Autodesk Inventor part; units mm, degrees
ref_plane "YZ Plane" through (0, 0, 0) normal (1, 0, 0) x (0, 1, 0)
ref_plane "XZ Plane" through (0, 0, 0) normal (0, 1, 0) x (-1, 0, 0)
ref_plane "XY Plane" through (0, 0, 0) normal (0, 0, 1) x (1, 0, 0)
sketch "Esquisse1" plane through (0, 0, 0) normal (0, 1, 0) x (-1, 0, 0)
  line L0 (-46.5, 50) -> (46.5, 50)
  line L1 (46.5, 50) -> (46.5, -50)
  line L2 (46.5, -50) -> (-46.5, -50)
  line L3 (-46.5, -50) -> (-46.5, 50)
  line L4 (-46.5, 50) -> (46.5, -50) construction
  line L5 (46.5, 50) -> (-46.5, -50) construction
  point P0 (0, 0)
  dimension "d0" = 100
  dimension "d1" = 93
extrude "Extrusion1" add sketch "Esquisse1" along normal blind 88
sketch "Esquisse2" plane through (0, 0, 0) normal (0, -1, 0) x (1, 0, 0)
  line L0 (-43.5, 47) -> (43.5, 47)
  line L1 (43.5, 47) -> (43.5, -47)
  line L2 (43.5, -47) -> (-43.5, -47)
  line L3 (-43.5, -47) -> (-43.5, 47)
  line L4 (-43.5, 47) -> (43.5, -47) construction
  line L5 (43.5, 47) -> (-43.5, -47) construction
  line L6 (46.5, 50) -> (46.5, -50)
  line L7 (-46.5, 50) -> (46.5, 50)
  point P0 (0, 0)
  dimension "d4" = 3
  dimension "d5" = 3
extrude "Extrusion2" cut sketch "Esquisse2" against normal blind 85
sketch "Esquisse3" plane through (-46.5, 0, 50) normal (0, 0, 1) x (1, 0, 0)
  line L0 (0, 88) -> (93, 88)
  line L1 (93, 88) -> (78, 88)
  line L2 (78, 88) -> (78, 73)
  line L3 (78, 73) -> (93, 73)
  line L4 (93, 73) -> (93, 88)
  point P0 (46.5, 0)
  dimension "d8" = 15
  dimension "d9" = 15
extrude "Extrusion3" cut sketch "Esquisse3" against normal up to surface (100 mm away)
sketch "Esquisse4" plane through (-46.5, 0, 50) normal (0, 0, 1) x (1, 0, 0)
  circle A0 centre (73, 68) radius 1.75
  circle A1 centre (33, 68) radius 1.75
  circle A2 centre (73, 30) radius 1.75
  circle A3 centre (33, 30) radius 1.75
  line L0 (93, 0) -> (93, 73)
  line L1 (0, 88) -> (78, 88)
  point P0 (46.5, 0)
  dimension "d12" = 40
  dimension "d13" = 3.5
  dimension "d14" = 3.5
  dimension "d15" = 3.5
  dimension "d16" = 3.5
  dimension "d17" = 40
  dimension "d18" = 0
  dimension "d19" = 0
  dimension "d20" = 38
  dimension "d21" = 20
  dimension "d22" = 20
  dimension "d23" = 0
extrude "Extrusion4" cut sketch "Esquisse4" against normal up to surface (3 mm away)
sketch "Esquisse5" plane through (46.5, 0, -50) normal (0, 0, -1) x (-1, 0, 0)
  circle A0 centre (66.8, 77) radius 2.1
  circle A1 centre (41.4, 77) radius 2.1
  circle A2 centre (11, 44.9) radius 2.1
  circle A3 centre (11, 7.4) radius 2.1
  line L0 (0, 0) -> (0, 73)
  line L1 (15, 88) -> (93, 88)
  line L2 (15, 88) -> (15, 73)
  line L3 (15, 73) -> (0, 73)
  circle A4 centre (83, 7.4) radius 2.1
  line L4 (93, 0) -> (93, 88)
  point P0 (46.5, 0)
  dimension "d26" = 4.2
  dimension "d27" = 4.2
  dimension "d28" = 4.2
  dimension "d29" = 4.2
  dimension "d30" = 11
  dimension "d31" = 0
  dimension "d32" = 11
  dimension "d33" = 0
  dimension "d34" = 37.5
  dimension "d35" = 25.4
  dimension "d36" = 26.4
  dimension "d37" = 28.1
  dimension "d38" = 4.2
  dimension "d39" = 0
  dimension "d40" = 10
extrude "Extrusion5" add sketch "Esquisse5" along normal blind 5.7
sketch "Esquisse6" plane through (-36.5, 7.4, -55.7) normal (0, 0, -1) x (-1, 0, 0)
  point P0 (-36.5, -7.4)
sketch "Esquisse7" plane through (-46.5, 0, 50) normal (0, 0, 1) x (1, 0, 0)
  line L0 (0, 88) -> (78, 88)
  line L1 (65, 88) -> (40, 88)
  line L2 (40, 88) -> (40, 79)
  line L3 (40, 79) -> (65, 79)
  line L4 (65, 79) -> (65, 88)
  line L5 (78, 73) -> (78, 88)
  point P0 (46.5, 0)
  point P1 (78, 80.5)
  point P2 (65, 83.5)
  dimension "d43" = 25
  dimension "d44" = 13
  dimension "d45" = 9
extrude "Extrusion6" cut sketch "Esquisse7" against normal up to surface (100 mm away)
sketch "Esquisse8" plane through (-20.3, 77, -55.7) normal (0, 0, -1) x (-1, 0, 0)
  line L0 (-13.8, 11) -> (26.2, 11)
  line L1 (-66.8, -77) -> (-66.8, -4)
  line L2 (26.2, 11) -> (-66.8, 11)
  line L3 (-66.8, 11) -> (-66.8, -77)
  line L4 (-66.8, -77) -> (26.2, -77)
  line L5 (26.2, -77) -> (26.2, 11)
  point P0 (-20.3, -77)
extrude "Extrusion7" cut sketch "Esquisse8" against normal up to surface (8.7 mm away)
sketch "Esquisse9" plane through (31.5, 88, -47) normal (0, 0, -1) x (-1, 0, 0)
  line L0 (13, 0) -> (0, 0)
  line L1 (13, -9) -> (13, -3)
  line L2 (0, 0) -> (13, 0)
  line L3 (13, 0) -> (13, -3)
  line L4 (13, -3) -> (0, -3)
  line L5 (0, -3) -> (0, 0)
  line L6 (78, -88) -> (78, 0)
  line L7 (75, -3) -> (38, -3)
  line L8 (78, 0) -> (68, 0)
  line L9 (68, 0) -> (68, -3)
  line L10 (68, -3) -> (78, -3)
  line L11 (78, -3) -> (78, 0)
  line L12 (75, -88) -> (75, -3)
  line L13 (78, -63) -> (75, -63)
  line L14 (75, -63) -> (75, -73)
  line L15 (75, -73) -> (78, -73)
  line L16 (78, -73) -> (78, -63)
  line L17 (78, -88) -> (75, -88)
  line L18 (-15, -88) -> (-15, -15)
  line L19 (-12, -88) -> (-12, -15)
  line L20 (-15, -38) -> (-12, -38)
  line L21 (-12, -38) -> (-12, -48)
  line L22 (-12, -48) -> (-15, -48)
  line L23 (-15, -48) -> (-15, -38)
  line L24 (-12, -88) -> (-15, -88)
  point P0 (31.5, -88)
  point P1 (-15, -48)
  dimension "d50" = 10
  dimension "d51" = 10
  dimension "d52" = 15
  dimension "d53" = 10
  dimension "d54" = 40
extrude "Extrusion8" cut sketch "Esquisse9" against normal blind 10 contours L3 L4 L5 L0 | L15 L12 L13 L6 | L10 L7 L9 L8 L6 | L18 L20 L19 L22
properties part number "support_imu_Impression 3D"
The model under review builds one solid part; all positions refer to its coordinate system, in mm. A direction names the side the tool comes from. Give positions to 0.01 mm unless a question says otherwise; leave off trailing zeros. Order: outer loops, then holes, each group sorted by start corner. A loop starts at its lowest first (then second) coordinate and runs counter-clockwise, first axis right, second up. Notation, with made-up numbers: (32, -5.5) -> (45, -5.5) arc R26 cw to (45, 15.5) -> close; hole circle Ø10 at (-16.5, 35). An arc over 180 degrees is marked (long way). Write item = value, one per line. Start each with the question number.
(1) Take a section at D-D (y = 47). Write out the cut boundary in (x, z).
(2) Take a section at C-C (z = -3.5). Write out the cut boundary in (x, y), plus the area to 3 significant figures.
(3) Draft analysis for pull direction X (two halves, no side actions). For faces 1 (the cylindrical face through (-13.88, 66.29, 48.52)), 2 (the cylindrical face through (24.75, 30.08, 48.52)), 3 (the flat face through (-36.5, 87, -42)), 4 (the flat face through (25, 85, 6)), state which applies: +X half, -X half, draft (parallel to the pull), parting line (faces both ways), or undercut.
(4) Tool access review of faces 5 (the flat face through (-41, 87, -37)), 6 (the flat face through (45, 50, -42)), 7 (the flat face through (-45, 15, -42)): name each direction out of +Z, -Z, +X, -X, +Y, -Y from which nothing blocks a thin tool from reaching the whole face with its end or side.
(5) For pin 1 Ø3.5 at (x, z) = (-44.5, -44) entering from +Y; pin 2 Ø10 at (y, z) = (84.5, 17.5) entering from +X; pin 3 Ø3.5 at (x, z) = (44.5, -43) entering from +Y, all flat-tipped, find the tip position at first contact; note any pin that passes through.
(6) Take a section at B-B (x = -13.5). Write out the cut boundary in (y, z), plus the area to 3 significant figures.
(7) Take a section at A-A (y = 68). Write out the cut boundary in (x, z).
(8) For L1, parallel to Y at x = -13.5, z = 47.6; L2, parallel to X at y = 5.5, z = -23; L3, parallel to X at y = 68, z = 48, list the stretches that pass through material, from the lowest coordinate up. Write a range as from..to.
Returned:
q1.outline = (-46.5, -47) -> (-43.5, -47) -> (-43.5, 47) -> (43.5, 47) -> (43.5, -37) -> (46.5, -37) -> (46.5, 50) -> (-46.5, 50) -> close
q2.outline = (-46.5, 0) -> (-43.5, 0) -> (-43.5, 85) -> (-6.5, 85) -> (-6.5, 88) -> (-46.5, 88) -> close; (18.5, 85) -> (31.5, 85) -> (31.5, 88) -> (18.5, 88) -> close; (43.5, 0) -> (46.5, 0) -> (46.5, 73) -> (43.5, 73) -> close
q2.area = 633 mm²
q3.face_1 = undercut
q3.face_2 = undercut
q3.face_3 = -X half
q3.face_4 = draft
q4.face_5 = -Z, -X, +Y
q4.face_6 = -Z, +X
q4.face_7 = -Z, -X
q5.pin_1 = 85
q5.pin_2 = 31.5
q5.pin_3 = 73
q6.outline = (0, 47) -> (28.25, 47) -> (28.25, 50) -> (0, 50) -> close; (31.75, 47) -> (66.25, 47) -> (66.25, 50) -> (31.75, 50) -> close; (69.75, 47) -> (85, 47) -> (85, -47) -> (88, -47) -> (88, 50) -> (69.75, 50) -> close
q6.area = 525 mm²
q7.outline = (-46.5, -47) -> (-43.5, -47) -> (-43.5, 47) -> (-15.25, 47) -> (-15.25, 50) -> (-46.5, 50) -> close; (-11.75, 47) -> (24.75, 47) -> (24.75, 50) -> (-11.75, 50) -> close; (28.25, 47) -> (43.5, 47) -> (43.5, -47) -> (46.5, -47) -> (46.5, 50) -> (28.25, 50) -> close
q8.L1 = 0..28.25, 31.75..66.25, 69.75..88
q8.L2 = -46.5..-43.5, 43.5..46.5
q8.L3 = -46.5..-15.25, -11.75..24.75, 28.25..46.5
